from build123d import *

# Parameters (mm, degrees)
F0_R     = 3
F1_DEPTH = 25
F2_DEPTH = 65
F4_DEPTH = 3


with BuildPart() as f1:
    # F0 (on Top) → F1 (new body)
    with BuildSketch(Plane.XY):
        with BuildLine():
            Line((7.5, -12.990381), (7.5, 12.990381))
            ThreePointArc((7.5, 12.990381), (0, 15), (-7.5, 12.990381))
            Line((-7.5, 12.990381), (-7.5, -12.990381))
            ThreePointArc((-7.5, -12.990381), (0, -15), (7.5, -12.990381))
        make_face()
        Circle(F0_R, mode=Mode.SUBTRACT)
    extrude(amount=F1_DEPTH)

    # F0 (on Top) → F2 (join)
    with BuildSketch(Plane.XY):
        Circle(F0_R)
    extrude(amount=F2_DEPTH)

    # F3 (on Right) → F4 (join, symmetric)
    with BuildSketch(Plane.YZ):
        Polygon((-12.5, 25), (0, 25), (0, 55), align=None)
    extrude(amount=F4_DEPTH, both=True)


solid = f1.part
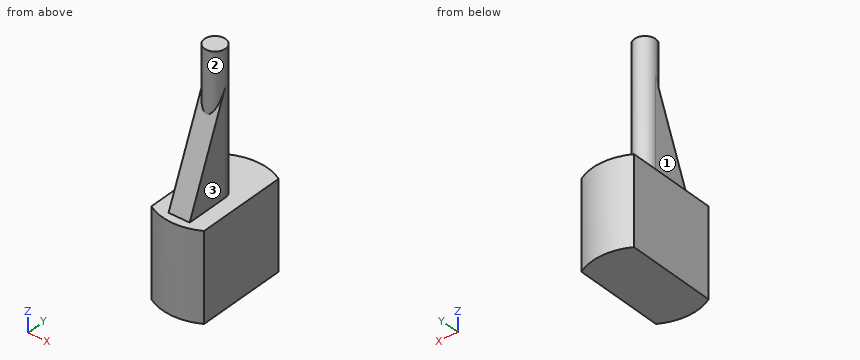
Verification items for the finished model (mm, model axes). Face numbers are marked on the shaded views. A direction names the side the tool comes from. Coordinates: 2 decimals unless noted, no trailing zeros. Loops run counter-clockwise (first coordinate to the right, second up) from the corner with the lowest first, then second, coordinate; pieces in that order, holes last. Notation, with made-up numbers: (34, 62) -> (59, 62) arc R15 cw to (59, 81) -> close; hole circle Ø9 at (88, 40.25). An arc over 180 degrees is marked (long way). Answer as a JSON object with one key per item and string values. Group by question number.
Item 1: Sectioned sample at C-C on z = 51.5. Record the boundary of the cut face in (x, y), plus the area to 3 significant figures.
Item 2: Scan lines: probe 1 along Z at (x, y) = (6.75, -12); probe 2 along Y at (x, z) = (-1, 48); probe 3 along Y at (x, z) = (6, 8.5). Record each from-to range of solid material in increasing order.
Item 3: Depth check by flat-ended pin: pin 1 (1 mm diameter, centred on x = 3, y = -9, fed in from -Z); pin 2 (14 mm diameter, centred on y = -3.5, z = 46.5, fed in from +X); pin 3 (2 mm diameter, centred on y = -2.5, z = 27.5, fed in from -X); pin 4 (4.5 mm diameter, centred on x = 2, y = -5.5, fed in from +Z). Enter the tip coordinate at first touch or a pass-through.
Item 4: Sectioned sample at D-D on z = 59. Record the boundary of the cut face in (x, y).
Item 5: Tool access check on the marked faces 1, 2 and 3. Record the directions out of +Z, -Z, +X, -X, +Y, -Y that give a thin tool (end or side, any length) a straight path to the whole face; none if there is none.
Item 6: Sectioned sample at B-B on x = 0. Record the boundary of the cut face in (y, z), plus the area to 3 significant figures.
Item 7: Sectioned sample at A-A on y = -9. Record the boundary of the cut face in (x, z), plus the area to 3 significant figures.
Evaluation:
{
 "1": {"outline": "(-3, -1.46) -> (-2.62, -1.46) arc R3 ccw to (2.62, -1.46) -> (3, -1.46) -> (3, 0) arc R3 ccw to (-3, 0) -> close", "area": "28.6 mm²"},
 "2": {"probe 1": "z = 0 to 25", "probe 2": "y = -2.92 to 2.83", "probe 3": "y = -13.75 to 13.75"},
 "3": {"pin 1": "stops at z = 0", "pin 2": "stops at x = 3", "pin 3": "stops at x = -3", "pin 4": "stops at z = 47.2"},
 "4": {"outline": "circle Ø6 at (0, 0)"},
 "5": {"face 1": "+Z, -X, +Y, -Y", "face 2": "+Z", "face 3": "+Z, +X, +Y, -Y"},
 "6": {"outline": "(-15, 0) -> (15, 0) -> (15, 25) -> (3, 25) -> (3, 65) -> (-3, 65) -> (-3, 47.8) -> (-12.5, 25) -> (-15, 25) -> close", "area": "1,100 mm²"},
 "7": {"outline": "(-7.5, 0) -> (7.5, 0) -> (7.5, 25) -> (3, 25) -> (3, 33.4) -> (-3, 33.4) -> (-3, 25) -> (-7.5, 25) -> close", "area": "425 mm²"}
}
